Geometry: final body of the model. Coordinates: model frame, mm. A direction names the side the tool comes from. Give positions to 0.01 mm unless a question says otherwise; leave off trailing zeros. Loops run counter-clockwise (first coordinate to the right, second up) from the corner with the lowest first, then second, coordinate; pieces in that order, holes last.
1. Section D-D, the plane z = 32.5. Output: boundary loops of the cut face in (x, y).
2. First-contact query: P1, Ø1.5, axis at x = -25.5, z = 7, coming from the -Y side; P2, Ø3, axis at x = 0, y = 13.38, coming from the -Z side; P3, Ø12, axis at x = -19, y = -27, coming from the -Z side; P4, Ø8, axis at x = 26, y = 0, coming from the +Z side. Flat tips, straight axial feed; report the tip coordinate or a pass-through.
3. Access query for faces 4 (the face through (-1, 9, 4)), 5 (the face through (0.325, -26.611, 26.767)). Directions: +Z, -Z, +X, -X, +Y, -Y. A direction counts if a zero-diameter tool reaches every point of the face in a straight line with its end or side. Return the directions, or none.
4. Section B-B, the plane x = -6.5. Output: boundary loops of the cut face in (y, z).
5. Section C-C, the plane y = 9. Output: boundary loops of the cut face in (x, z), then the cut area to 3 significant figures.
6. Material intervals for line 1 along Y through (x, z) = (-9, 29); line 2 along Z through (x, y) = (9, -12.5); line 3 along Y through (x, z) = (26, 1.4), sorted ascending.
7. Draft query along X for faces 1 (the face through (27.31, 14.38, 2.03)), 2 (the face through (36, -19, 16)), 3 (the face through (1, 1, 0)). Return one class per face: +X half, -X half, draft (parallel to the pull), parting line (faces both ways), or undercut.
8. Section A-A, the plane x = -26. Output: boundary loops of the cut face in (y, z), then the cut area to 3 significant figures.
from build123d import *

# Parameters (mm, degrees)
F0_W     = 72
F0_H     = 45
F1_DEPTH = 4
F2_D     = 3.3
F2_DEPTH = 8
F2_TIP   = 0.9914200214
F4_DEPTH = 72
F5_R     = 15
F7_D     = 3
F7_DEPTH = 25
F7_TIP   = 0.9012909285


with BuildPart() as f1:
    # F0 (on Top) → F1 (new body)
    with BuildSketch(Plane.XY):
        Rectangle(F0_W, F0_H)
    extrude(amount=F1_DEPTH)

    # F2
    with Locations(Plane(origin=(0, 0, 0), x_dir=(1, 0, 0), z_dir=(0, 0, -1))):
        with Locations((-26, -13.3780119941), (0, -13.3780119941), (26, -13.3780119941)):
            Hole(F2_D / 2, depth=F2_DEPTH)
            with Locations((0, 0, -(F2_DEPTH + F2_TIP / 2))):  # 118° drill point
                Cone(0, F2_D / 2, F2_TIP, mode=Mode.SUBTRACT)

    # F3 (on face) → F4 (join)
    with BuildSketch(Plane.YZ.offset(36)):
        Polygon((-22.5, 4), (-9.5828315243, 4), (-24.3840366602, 41.4623506367), (-35.0105427206, 41.4623506367), (-35.0105427206, 0), (-22.5, 0), align=None)
    extrude(amount=-F4_DEPTH)

    # F5
    f5_edges = [f1.edges().sort_by_distance(p)[0] for p in [
        (0, -35.010543, 0),
        (0, -9.582832, 4),
    ]]
    fillet(f5_edges, radius=F5_R)

    # F7
    with Locations(Plane.XZ.offset(35.0105427206)):
        with Locations((-20.9683738649, 28.2311753184), (20.9683738649, 28.2311753184), (0, 28.2311753184)):
            Hole(F7_D / 2, depth=F7_DEPTH)
            with Locations((0, 0, -(F7_DEPTH + F7_TIP / 2))):  # 118° drill point
                Cone(0, F7_D / 2, F7_TIP, mode=Mode.SUBTRACT)


solid = f1.part
Answers below:
1. outline: (-36, -35.01) - (36, -35.01) - (36, -20.84) - (-36, -20.84) - close
2. P1: stops at y = -33.14
2. P2: passes through
2. P3: stops at z = 0.03
2. P4: stops at z = 4.73
3. face 4: +Z, +X, -X, +Y
3. face 5: +Y, -Y
4. outline: (-35.01, 15) arc R15 ccw to (-20.01, 0) - (22.5, 0) - (22.5, 4) - (0.62, 4) arc R15 cw to (-13.33, 13.49) - (-24.38, 41.46) - (-35.01, 41.46) - close
5. outline: (-36, 0) - (36, 0) - (36, 4) - (-36, 4) - close
5. area: 288 mm2
6. line 1: y = -35.01 to -19.46
6. line 2: z = 0 to 11.73
6. line 3: y = -26.34 to 11.73, 15.03 to 22.5
7. face 1: undercut
7. face 2: +X half
7. face 3: draft
8. outline: (-35.01, 15) arc R15 ccw to (-20.01, 0) - (11.73, 0) - (11.73, 4) - (0.62, 4) arc R15 cw to (-13.33, 13.49) - (-24.38, 41.46) - (-35.01, 41.46) - close; (15.03, 0) - (22.5, 0) - (22.5, 4) - (15.03, 4) - close
8. area: 863 mm2
